Input: dimensioned drawing with shaded views. Units: mm. Origin: part minimum x, y, z. Round coordinates to 2 decimals unless told otherwise and drop trailing zeros. Write each loop counter-clockwise with the first axis right and the second up, starting at its lowest first coordinate (ties: lowest second). Pieces come first, ordered by that corner, then holes. Notation, with made-up numbers: M -17,88.5 L 17,88.5 A13 cw 17,97.5 Z; hole C 87.5,-5 d1. An arc over 180 degrees is marked long. Put each result on its own line as item: value. Start each with the question number.
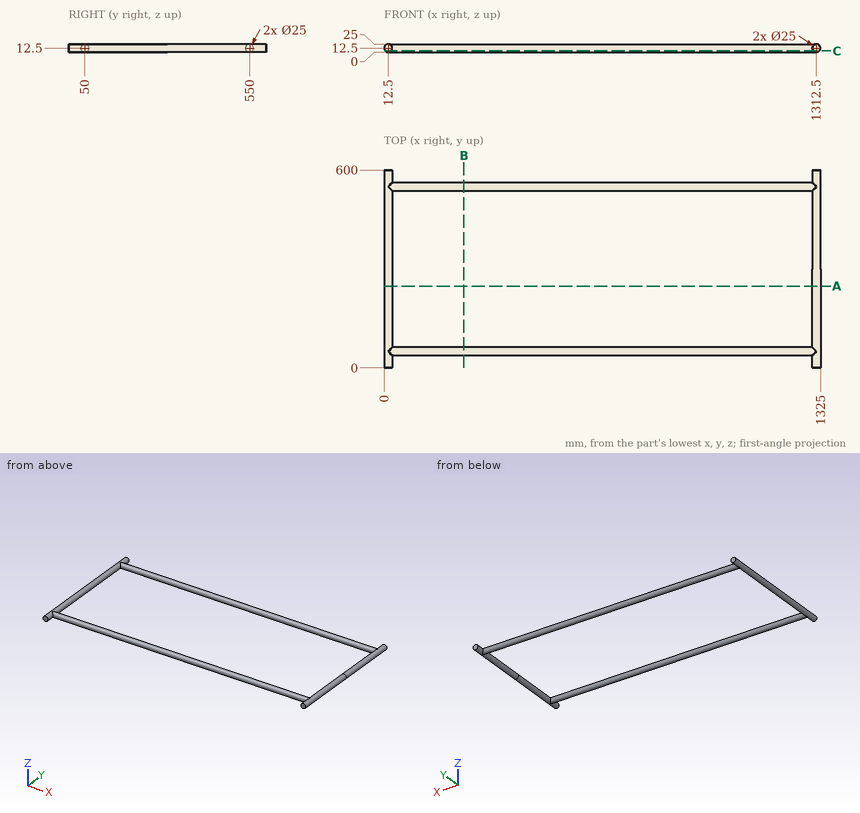
1) Section B-B, the plane x = 242.5. Output: boundary loops of the cut face in (y, z), and give its area (3 significant figures).
2) Section A-A, the plane y = 248.5. Output: boundary loops of the cut face in (x, z).
3) First-contact query: pin 1 (10 mm diameter, centred on y = 372.5, z = 9.5, fed in from -X); pin 2 (3 mm diameter, centred on y = 173, z = 18.5, fed in from -X); pin 3 (1 mm diameter, centred on x = 1127.5, z = 19.5, fed in from +Y); pin 4 (1 mm diameter, centred on x = 172.5, z = 4, fed in from +Y). Flat tips, straight axial feed; report the tip coordinate or a pass-through.
4) Section C-C, the plane z = 4. Output: boundary loops of the cut face in (x, y), and give its area (3 significant figures).
5) Ray query, probe 1 along Y at (x, z) = (1067.5, 13.5); probe 2 along X at (y, z) = (175, 13.5); probe 3 along X at (y, z) = (357, 8). Return the intervals inside material, ascending.
Solved:
1. outline: C 50,12.5 d25; C 550,12.5 d25
1. area: 982 mm2
2. outline: C 12.5,12.5 d25; C 1312.5,12.5 d25
3. pin 1: stops at x = 0
3. pin 2: stops at x = 0.84
3. pin 3: stops at y = 560.68
3. pin 4: stops at y = 559.6
4. outline: M 3.33,0 L 21.67,0 L 21.67,40.83 L 1303.33,40.83 L 1303.33,0 L 1321.67,0 L 1321.67,600 L 1303.33,600 L 1303.33,559.17 L 21.67,559.17 L 21.67,600 L 3.33,600 Z; hole M 21.67,59.17 L 1303.33,59.17 L 1303.33,540.83 L 21.67,540.83 Z
4. area: 69,000 mm2
5. probe 1: y = 37.54 to 62.46, 537.54 to 562.46
5. probe 2: x = 0.04 to 24.96, 1300.04 to 1324.96
5. probe 3: x = 0.84 to 24.16, 1300.84 to 1324.16
